from build123d import *

# Parameters (mm, degrees)
PAD_DEPTH           = 2.15
PAD_DEPTH_BACK      = 5.4
SKETCH001_W         = 0.5
SKETCH001_H         = 0.3
PAD001_DEPTH        = 0.6
PAD001_DEPTH_BACK   = 4.1
LINEARPATTERN_COUNT = 3
LINEARPATTERN_PITCH = 2.54


with BuildPart() as part:
    # Sketch → Pad (new body, two sides)
    with BuildSketch(Plane.XZ) as pad_sk:
        Polygon((-2.76, 0.5), (7.84, 0.5), (7.84, 0), (8.34, 0), (8.34, 10.2), (-3.26, 10.2), (-3.26, 0), (-2.76, 0), align=None)
    extrude(amount=PAD_DEPTH)
    extrude(pad_sk.sketch, amount=-PAD_DEPTH_BACK)

    # Sketch001 → Pad001 (join, two sides)
    with BuildSketch(Plane.XY) as pad001_sk:
        Rectangle(SKETCH001_W, SKETCH001_H)
    pad001 = extrude(amount=PAD001_DEPTH) + extrude(pad001_sk.sketch, amount=-PAD001_DEPTH_BACK)

    # LinearPattern: Pad001 ×3
    with Locations(*[(i * LINEARPATTERN_PITCH, 0, 0) for i in range(1, LINEARPATTERN_COUNT)]):
        add(pad001)


solid = part.part
Read the model definition and answer for the solid it produces. Units are mm, in the model's axes. Coordinates: 2 decimals unless noted, no trailing zeros. Loops run counter-clockwise (first coordinate to the right, second up) from the corner with the lowest first, then second, coordinate; pieces in that order, holes last.
Q1. The mould has two halves that part along X. Classify faces 1 (the face through (2, -2.15, 5)), 2 (the face through (-3.26, 2, 5)), 3 (the face through (2, 2, 0.5)), 4 (the face through (8.34, 2, 5)): +X half, -X half, draft (parallel to the pull), parting line (faces both ways), or undercut.
Q2. Each of these flat-tipped pins is pushed along its axis until it touches: pin 1 Ø0.6 at (x, z) = (5, -2) entering from -Y; pin 2 Ø0.6 at (x, z) = (5, -1) entering from +Y; pin 3 Ø2.5 at (x, y) = (4, 0) entering from -Z. Where does it stop, or does it pass through?
Q3. The part is cut by section C-C on x = -0.5. Write down the section's boundary in (y, z), and give its area (3 significant figures).
Q4. Consider probe 1 along Z at (x, y) = (5, 0.75); probe 2 along Y at (x, z) = (5.25, -3). Determine where each line is inside the solid, lowest interval first.
Q5. The part is cut by section A-A on x = 5. Write down the section's boundary in (y, z), and give its area (3 significant figures).
Q6. The part is cut by section B-B on y = 3. Write down the section's boundary in (x, z).
Results below:
1. face 1: draft
1. face 2: -X half
1. face 3: undercut
1. face 4: +X half
2. pin 1: stops at y = -0.15
2. pin 2: stops at y = 0.15
2. pin 3: stops at z = -4.1
3. outline: (-2.15, 0.5) - (5.4, 0.5) - (5.4, 10.2) - (-2.15, 10.2) - close
3. area: 73.2 mm2
4. probe 1: z = 0.5 to 10.2
4. probe 2: y = -0.15 to 0.15
5. outline: (-2.15, 0.5) - (-0.15, 0.5) - (-0.15, -4.1) - (0.15, -4.1) - (0.15, 0.5) - (5.4, 0.5) - (5.4, 10.2) - (-2.15, 10.2) - close
5. area: 74.6 mm2
6. outline: (-3.26, 0) - (-2.76, 0) - (-2.76, 0.5) - (7.84, 0.5) - (7.84, 0) - (8.34, 0) - (8.34, 10.2) - (-3.26, 10.2) - close
